Part model, mm, in its own coordinate system. A direction names the side the tool comes from. Give positions to 0.01 mm unless a question says otherwise; leave off trailing zeros. Loops run counter-clockwise (first coordinate to the right, second up) from the corner with the lowest first, then second, coordinate; pieces in that order, holes last. Notation, with made-up numbers: M 55.5,89.25 L 87.5,89.25 A26 cw 87.5,108.25 Z; hole C 12,-17.5 d11. An arc over 180 degrees is marked long. Answer in a Markdown table with one row per item.
Autodesk Inventor part; units mm, degrees
ref_plane "YZ Plane" through (0, 0, 0) normal (1, 0, 0) x (0, 1, 0)
ref_plane "XZ Plane" through (0, 0, 0) normal (0, 1, 0) x (-1, 0, 0)
ref_plane "XY Plane" through (0, 0, 0) normal (0, 0, 1) x (1, 0, 0)
sketch "Sketch1" plane through (0, 0, 0) normal (0, 0, 1) x (1, 0, 0)
  line L0 (0, 0) -> (25, 0)
  line L1 (25, 0) -> (25, 40)
  line L2 (25, 40) -> (0, 40)
  line L3 (0, 40) -> (0, 0)
  dimension "d1" = 25
  dimension "d2" = 40
  dimension "d3" = 25
extrude "Extrusion1" add sketch "Sketch1" against normal blind 30
sketch "Sketch2" plane through (25, 0, 0) normal (1, 0, 0) x (0, 0, -1)
  line L0 (0, 0) -> (30, 0)
  circle A0 centre (15, 6.56) radius 2.46
extrude "Extrusion2" cut sketch "Sketch2" against normal blind 30
sketch "Sketch3" plane through (0, 0, 0) normal (-1, 0, 0) x (0, 0, 1)
  line L0 (0, 0) -> (-30, 0)
  line L1 (-25.05, 0) -> (-4.95, 0)
  line L2 (-4.95, 0) -> (-4.95, 33.12)
  line L3 (-4.95, 33.12) -> (-25.05, 33.12)
  line L4 (-25.05, 33.12) -> (-25.05, 0)
  dimension "d11" = 20.1
extrude "Extrusion3" cut sketch "Sketch3" against normal blind 20
sketch "Sketch4" plane through (0, 0, 0) normal (0, -1, 0) x (1, 0, 0)
  line L0 (20, -4.95) -> (20, -25.05)
  line L1 (20, -15) -> (25, -15)
  line L2 (25, 0) -> (25, -30)
  line L3 (20, -8.025) -> (25, -8.025)
  line L4 (25, -8.025) -> (25, -21.975)
  line L5 (25, -21.975) -> (20, -21.975)
  line L6 (20, -21.975) -> (20, -8.025)
  line L7 (20, -8.025) -> (25, -21.975) construction
  line L8 (25, -8.025) -> (20, -21.975) construction
  line L9 (25, -12.54) -> (25, -17.46)
  point P0 (0, 0)
  point P1 (22.5, -15)
  dimension "d14" = 13.95
extrude "Extrusion4" add sketch "Sketch4" along normal blind 15
sketch "Sketch5" plane through (20, 0, 0) normal (-1, 0, 0) x (0, 0, 1)
  circle A0 centre (-15, 6.56) radius 2.46
  circle A1 centre (-15, 6.56) radius 4.7025
  circle A2 centre (-15, 6.56) radius 2.46
  circle A3 centre (-15, 6.56) radius 2.46
  point P0 (0, 0)
  dimension "d17" = 9.405
extrude "Extrusion5" cut sketch "Sketch5" against normal blind 2.1
sketch "Sketch6" plane through (25, 0, 0) normal (1, 0, 0) x (0, 0, -1)
  circle A0 centre (15, 6.56) radius 4.7025
  line L0 (15, 6.56) -> (15, 23.56)
  circle A1 centre (15, 23.56) radius 2.46
  point P0 (0, 0)
  dimension "d20" = 17
  dimension "d21" = 4.92
extrude "Extrusion6" cut sketch "Sketch6" against normal blind 10 contours A1
sketch "Sketch7" plane through (20, 0, 0) normal (-1, 0, 0) x (0, 0, 1)
  circle A0 centre (-15, 23.56) radius 2.46
  circle A1 centre (-15, 23.56) radius 4.7025
  point P0 (0, 0)
  dimension "d24" = 9.405
extrude "Extrusion7" cut sketch "Sketch7" against normal blind 2.1
sketch "Sketch9" plane through (25, 0, 0) normal (1, 0, 0) x (0, 0, -1)
  circle A0 centre (15, 6.56) radius 2.46
  circle A1 centre (15, 6.56) radius 2.46
  circle A2 centre (15, 23.56) radius 2.46
  circle A3 centre (15, 23.56) radius 2.46
  line L0 (30, 40) -> (30, 0)
  line L1 (30, 0) -> (30, 40)
  line L2 (30, 40) -> (0, 40)
  line L3 (0, 40) -> (0, 0)
  line L4 (0, 0) -> (8.025, 0)
  line L5 (21.975, 0) -> (21.975, -15)
  line L6 (21.975, -15) -> (8.025, -15)
  line L7 (8.025, -15) -> (8.025, 0)
  line L8 (0, 0) -> (8.025, 0)
  line L9 (21.975, 0) -> (30, 0)
extrude "Extrusion8" add sketch "Sketch9" along normal blind 5
sketch "Sketch10" plane through (0, 40, 0) normal (0, 1, 0) x (1, 0, 0)
  line L0 (0, 30) -> (30, 30)
  line L1 (30, 0) -> (0, 0)
  line L2 (0, 30) -> (30, 30)
  line L3 (30, 30) -> (30, 0)
  line L4 (30, 0) -> (0, 0)
  line L5 (0, 0) -> (0, 30)
extrude "Extrusion9" add sketch "Sketch10" along normal blind 30
sketch "Sketch12" plane through (30, 0, 0) normal (1, 0, 0) x (0, 0, -1)
  circle A0 centre (15, 6.56) radius 2.46
  line L0 (15, 6.56) -> (15, 15.06)
  circle A1 centre (15, 15.06) radius 2.525
  point P0 (0, 0)
  dimension "d31" = 8.5
  dimension "d33" = 5.05
extrude "Extrusion10" cut sketch "Sketch12" against normal blind 30 contours A1
sketch "Sketch14" plane through (0, 0, 0) normal (0, 0, 1) x (1, 0, 0)
  line L0 (30, 70) -> (0, 70)
  line L1 (0, 70) -> (0, 85)
  line L2 (30, 0) -> (30, 70)
  line L3 (30, 118) -> (30, 70)
  line L4 (30, 105) -> (30, 100)
  line L5 (-7, 134) -> (-12, 136)
  line L6 (-7, 102) -> (-12, 100)
  line L7 (-7, 102) -> (-2, 118)
  line L8 (-2, 118) -> (-7, 134)
  line L9 (15, 136) -> (30, 118)
  line L10 (-12, 136) -> (15, 136)
  line L11 (0, 85) -> (0, 100)
  line L12 (0, 100) -> (-12, 100)
  point P0 (0, 0)
  dimension "d82" = 12
extrude "Extrusion12" add sketch "Sketch14" against normal blind 30
sketch "Sketch15" plane through (0, 0, -25.05) normal (-1, 0, 0) x (0, 0, 1)
  line L0 (0, 33.12) -> (20.1, 33.12)
  line L1 (20.1, 33.12) -> (20.1, 0)
  line L2 (0, 33.12) -> (20.1, 33.12)
  line L3 (20.1, 33.12) -> (20.1, 31.1)
  line L4 (20.1, 31.1) -> (0, 31.1)
  line L5 (0, 31.1) -> (0, 33.12)
  point P0 (25.05, 0)
  dimension "d57" = 2.02
extrude "Extrusion13" add sketch "Sketch15" against normal blind 20
properties part number "rec_a_32mm_x_30mm"
(1) Saw through at C-C (x = 2). Write the cut outline in (y, z), plus the area to 3 significant figures.
Recorded:
| item | result |
|---|---|
| outline | M 0,-30 L 136,-30 L 136,0 L 0,0 L 0,-4.95 L 31.1,-4.95 L 31.1,-25.05 L 0,-25.05 Z |
| area | 3,450 mm^2 |
(2) Which spindle directions (+Z, -Z, +X, -X, +Y, -Y) get a long thin tool onto all of the face, cutting with end or side? Do faces 1 (the face through (18, 0, -27)), 2 (the face through (-4.465, 125.888, -14.79)), 3 (the face through (0, 62, -15)), 4 (the face through (25, -8, -8.025)), 5 (the face through (10, 31.1, -15)). Say none if no direction does.
Recorded:
| item | result |
|---|---|
| face 1 | -Z, +X, -X, -Y |
| face 2 | +Z, -Z, -X |
| face 3 | +Z, -Z, -X, -Y |
| face 4 | +Z, +X, -X, -Y |
| face 5 | -X, -Y |
(3) Saw through at D-D (z = -2.5). Write the cut outline in (x, y), plus the area to 3 significant figures.
Recorded:
| item | result |
|---|---|
| outline | M -12,100 L 0,100 L 0,0 L 30,0 L 30,118 L 15,136 L -12,136 L -7,134 L -2,118 L -7,102 Z |
| area | 4,130 mm^2 |
(4) Saw through at B-B (z = -15). Give the number of separate pieces and of enclosed holes in the cut face, plus the area to 3 significant figures.
Recorded:
| item | result |
|---|---|
| separate pieces | 4 |
| enclosed holes | 0 |
| area | 3,490 mm^2 |
(5) Pin check, flat tips, straight feed: pin 1 Ø10 at (y, z) = (67.5, -26.5) entering from -X; pin 2 Ø3.5 at (x, z) = (-7.5, -16.5) entering from -Y; pin 3 Ø10 at (x, z) = (8, -15.5) entering from -Y. Stop position of each tip, or through.
Recorded:
| item | result |
|---|---|
| pin 1 | stops at x = 0 |
| pin 2 | stops at y = 100 |
| pin 3 | stops at y = 31.1 |
(6) Saw through at A-A (y = 15.06). Write the cut outline in (x, z) (3 decimals), plus the area to 4 significant figures.
Recorded:
| item | result |
|---|---|
| outline | M 0,-30 L 30,-30 L 30,-17.525 L 20,-17.525 L 20,-25.05 L 0,-25.05 Z; M 0,-4.95 L 20,-4.95 L 20,-12.475 L 30,-12.475 L 30,0 L 0,0 Z |
| area | 447.5 mm^2 |
(7) Drill centre lines: line 1 along Z through (x, y) = (25.75, 23.56); line 2 along Y through (x, z) = (27.25, -15) (3 decimals); line 3 along Y through (x, z) = (26, -15) (3 decimals). Where is each one in solid material? Low to high.
Recorded:
| item | result |
|---|---|
| line 1 | z = -30 to -17.46, -12.54 to 0 |
| line 2 | y = -15 to 4.1, 9.02 to 12.535, 17.585 to 21.1, 26.02 to 121.3 |
| line 3 | y = -15 to 4.1, 9.02 to 12.535, 17.585 to 21.1, 26.02 to 122.8 |
(8) Pull direction Y, two halves, no side cores. Call faces 6 (the face through (1, 136, -15)), 7 (the face through (10, 16, -25.05)), 8 (the face through (25.07, 15.171, -12.477)): +Y half, -Y half, draft (parallel to the pull), parting line (faces both ways), or undercut.
Recorded:
| item | result |
|---|---|
| face 6 | +Y half |
| face 7 | draft |
| face 8 | undercut |
